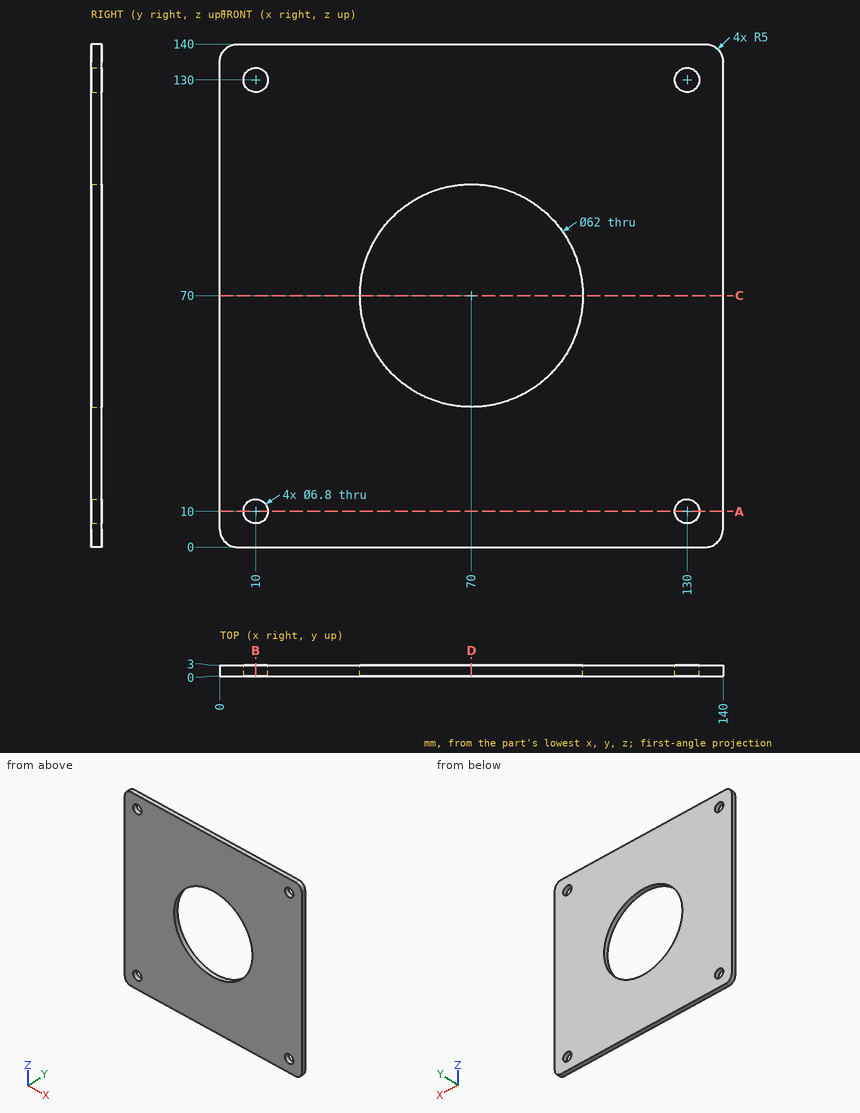
Here's the drawing with two shaded views (mm, measured from the low corner). I have some questions. Give positions to 0.01 mm unless a question says otherwise; leave off trailing zeros. Write each loop counter-clockwise with the first axis right and the second up, starting at its lowest first coordinate (ties: lowest second). Pieces come first, ordered by that corner, then holes. Notation, with made-up numbers: (37, 3.25) - (92, 3.25) arc R10 ccw to (92, 11.25) - close; hole circle Ø7 at (18.25, 84.5). An arc over 180 degrees is marked (long way). Write item = value, one per line. Start each with the question number.
1. Imagine slicing it at C-C (z = 70). Please give me the cut outline in (x, y), and give its area (3 significant figures).
2. Please list where these lines run through material, in increasing order: line 1 (X direction, y = 0.6, z = 130); line 2 (X direction, y = 1.75, z = 8).
3. For pin 1 (4 mm diameter, centred on x = 130, z = 10, fed in from +Y), with a flat end and sliding along its axis, tell me the tip position at first contact or that it passes through.
4. Imagine slicing it at B-B (x = 10). Please give me the cut outline in (y, z).
5. Imagine slicing it at D-D (x = 70). Please give me the cut outline in (y, z).
6. Imagine slicing it at A-A (z = 10). Please give me the cut outline in (x, y), and give its area (3 significant figures).
Worked answers:
q1.outline = (0, 0) - (39, 0) - (39, 3) - (0, 3) - close; (101, 0) - (140, 0) - (140, 3) - (101, 3) - close
q1.area = 234 mm2
q2.line_1 = 0 to 6.6, 13.4 to 126.6, 133.4 to 140
q2.line_2 = 0 to 7.25, 12.75 to 127.25, 132.75 to 140
q3.pin_1 = through
q4.outline = (0, 0) - (3, 0) - (3, 6.6) - (0, 6.6) - close; (0, 13.4) - (3, 13.4) - (3, 126.6) - (0, 126.6) - close; (0, 133.4) - (3, 133.4) - (3, 140) - (0, 140) - close
q5.outline = (0, 0) - (3, 0) - (3, 39) - (0, 39) - close; (0, 101) - (3, 101) - (3, 140) - (0, 140) - close
q6.outline = (0, 0) - (6.6, 0) - (6.6, 3) - (0, 3) - close; (13.4, 0) - (126.6, 0) - (126.6, 3) - (13.4, 3) - close; (133.4, 0) - (140, 0) - (140, 3) - (133.4, 3) - close
q6.area = 379 mm2
